Model file for the job. Use its own axes, mm. A direction names the side the tool comes from. Round coordinates to 2 decimals unless told otherwise and drop trailing zeros. Write each loop counter-clockwise with the first axis right and the second up, starting at its lowest first coordinate (ties: lowest second). Pieces come first, ordered by that corner, then holes. Notation, with made-up numbers: (-31, 62) - (19, 62) arc R21 ccw to (19, 77) - close; hole circle Ø9 at (-6, 36.25). An arc over 180 degrees is marked (long way). One line per item, written item: value.
Autodesk Inventor part; units mm, degrees
ref_plane "YZ Plane" through (0, 0, 0) normal (1, 0, 0) x (0, 1, 0)
ref_plane "XZ Plane" through (0, 0, 0) normal (0, 1, 0) x (-1, 0, 0)
ref_plane "XY Plane" through (0, 0, 0) normal (0, 0, 1) x (1, 0, 0)
sketch "Sketch1" plane through (0, 0, 0) normal (1, 0, 0) x (0, 1, 0)
  line L0 (40, 12.5) -> (-40, 12.5)
  line L1 (-40, 12.5) -> (-40, -12.5)
  line L2 (-40, -12.5) -> (40, -12.5)
  line L3 (40, -12.5) -> (40, 12.5)
  line L4 (40, 12.5) -> (-40, -12.5) construction
  line L5 (-40, 12.5) -> (40, -12.5) construction
  point P0 (0, 0)
  dimension "d0" = 80
  dimension "d1" = 25
extrude "Extrusion1" add sketch "Sketch1" along normal mid plane 600
sketch "Sketch2" plane through (-300, -40, 12.5) normal (0, 0, 1) x (1, 0, 0)
  circle A0 centre (300, 40) radius 20
  point P0 (300, 40)
  dimension "d4" = 40
extrude "Extrusion2" cut sketch "Sketch2" against normal up to next
sketch "Sketch3" plane through (0, 0, 0) normal (1, 0, 0) x (0, 1, 0)
  line L0 (-25, -20) -> (25, -20)
  line L1 (25, -20) -> (25, -5)
  line L2 (25, -5) -> (-25, -5)
  line L3 (-25, -5) -> (-25, -20)
  line L4 (40, -12.5) -> (-40, -12.5)
  line L5 (-25, -20) -> (25, -5) construction
  line L6 (25, -20) -> (-25, -5) construction
  line L7 (20, 12.5) -> (20, -12.5)
  line L8 (-40, 12.5) -> (40, 12.5)
  line L9 (-25, 20) -> (25, 20)
  line L10 (25, 20) -> (25, 5)
  line L11 (25, 5) -> (-25, 5)
  line L12 (-25, 5) -> (-25, 20)
  line L13 (40, 12.5) -> (-40, 12.5)
  line L14 (-25, 20) -> (25, 5) construction
  line L15 (25, 20) -> (-25, 5) construction
  point P0 (0, -12.5)
  point P1 (20, 5)
  point P2 (0, 12.5)
  dimension "d10" = 50
  dimension "d11" = 15
  dimension "d15" = 15
extrude "Extrusion3" cut sketch "Sketch3" along normal mid plane 550
properties part number "spiritLevel"
1. Band-saw the part on A-A on x = 0. Write the cut outline in (y, z), plus the area to 3 significant figures.
Report:
outline: (-40, -12.5) - (-25, -12.5) - (-25, -5) - (-20, -5) - (-20, 5) - (-25, 5) - (-25, 12.5) - (-40, 12.5) - close; (20, -5) - (25, -5) - (25, -12.5) - (40, -12.5) - (40, 12.5) - (25, 12.5) - (25, 5) - (20, 5) - close
area: 850 mm²
2. Band-saw the part on D-D on z = 0.5. Write the cut outline in (x, y).
Report:
outline: (-300, -40) - (300, -40) - (300, 40) - (-300, 40) - close; hole circle Ø40 at (0, 0)
3. Band-saw the part on B-B on y = 0. Write the cut outline in (x, z), plus the area to 3 significant figures.
Report:
outline: (-300, -12.5) - (-275, -12.5) - (-275, -5) - (-20, -5) - (-20, 5) - (-275, 5) - (-275, 12.5) - (-300, 12.5) - close; (20, -5) - (275, -5) - (275, -12.5) - (300, -12.5) - (300, 12.5) - (275, 12.5) - (275, 5) - (20, 5) - close
area: 6,350 mm²
4. Tool access for faces 1 (the face through (-4, 23, 5)), 2 (the face through (-4, 23, -5)), 3 (the face through (-4, -40, 0)): list every direction of +Z, -Z, +X, -X, +Y, -Y with a clear straight run to the whole face (end or side of a thin tool).
Report:
face 1: +Z
face 2: -Z
face 3: +Z, -Z, +X, -X, -Y
5. Band-saw the part on C-C on x = -184. Write the cut outline in (y, z).
Report:
outline: (-40, -12.5) - (-25, -12.5) - (-25, -5) - (25, -5) - (25, -12.5) - (40, -12.5) - (40, 12.5) - (25, 12.5) - (25, 5) - (-25, 5) - (-25, 12.5) - (-40, 12.5) - close
6. Drop flat-ended pins along their axis: pin 1 (4 mm diameter, centred on x = -201, y = 20.5, fed in from +Z); pin 2 (8 mm diameter, centred on x = 150.5, y = -8.5, fed in from -Z). Give the stop position or say it passes through.
Report:
pin 1: z = 5
pin 2: z = -5
7. Wall check: probe 1 along Y at (x, z) = (-225, -9); probe 2 along Y at (x, z) = (0, -3); probe 3 along Z at (x, y) = (-165.5, 2). Give the ranges that are in metal, low to high. Write a range as [from, to].
Report:
probe 1: [-40, -25], [25, 40]
probe 2: [-40, -20], [20, 40]
probe 3: [-5, 5]
8. Mould opens along Y. For faces 4 (the face through (-4, 40, 0)), 5 (the face through (-4.336, -19.524, 0.07)), 6 (the face through (-4, 27, 12.5)) say: released by +Y, released by -Y, zero draft, split by the parting line, or undercut.
Report:
face 4: released by +Y
face 5: undercut
face 6: zero draft
